CAD build for the part. Positions are in the model's coordinates, mm. Give positions to 0.01 mm unless a question says otherwise; leave off trailing zeros. Loops run counter-clockwise (first coordinate to the right, second up) from the corner with the lowest first, then second, coordinate; pieces in that order, holes last. Notation, with made-up numbers: M 71.25,37 L 87.25,37 A25 cw 87.25,73 Z; hole C 18.5,-18 d8. An arc over 180 degrees is marked long. Answer as CSV lines item,"result".
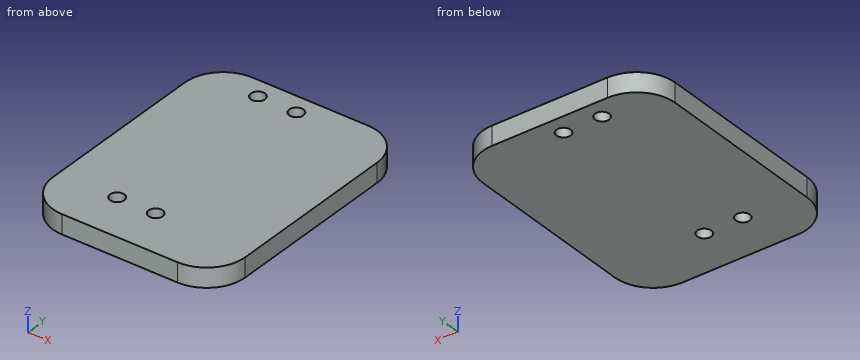
from build123d import *

# Parameters (mm, degrees)
ESQUISSE1_W             = 50
ESQUISSE1_H             = 65
BOSS_EXTRU_1_DEPTH      = 5
ESQUISSE2_R             = 1.85
ENL_V_MAT_EXTRU_1_DEPTH = 42.306779105
CONG_1_R                = 10


with BuildPart() as part:
    # Esquisse1 → Boss.-Extru.1 (new body)
    with BuildSketch(Plane.XY):
        Rectangle(ESQUISSE1_W, ESQUISSE1_H)
    extrude(amount=BOSS_EXTRU_1_DEPTH)

    # Esquisse2 → Enlèv. mat.-Extru.1 (cut, through all)
    with BuildSketch(Plane.XY.offset(5)):
        with Locations((-9.8, -20.5)):
            Circle(ESQUISSE2_R)
        with Locations((0.2, -20.5)):
            Circle(ESQUISSE2_R)
        with Locations((-9.8, 27.5)):
            Circle(ESQUISSE2_R)
        with Locations((0.2, 27.5)):
            Circle(ESQUISSE2_R)
    extrude(amount=-ENL_V_MAT_EXTRU_1_DEPTH, mode=Mode.SUBTRACT)

    # Congé1
    cong_1_edges = [part.edges().sort_by_distance(p)[0] for p in [
        (25, -32.5, 2.5),
        (-25, -32.5, 2.5),
        (-25, 32.5, 2.5),
        (25, 32.5, 2.5),
    ]]
    fillet(cong_1_edges, radius=CONG_1_R)


solid = part.part
1) Band-saw the part on C-C on z = 4.15. Give the cut face in (x, y), and give its area (3 significant figures).
Answer below:
outline,"M -25,-22.5 A10 ccw -15,-32.5 L 15,-32.5 A10 ccw 25,-22.5 L 25,22.5 A10 ccw 15,32.5 L -15,32.5 A10 ccw -25,22.5 Z; hole C -9.8,-20.5 d3.7; hole C -9.8,27.5 d3.7; hole C 0.2,-20.5 d3.7; hole C 0.2,27.5 d3.7"
area,"3,120 mm^2"
2) Band-saw the part on B-B on y = -20.5. Give the cut face in (x, z), and give its area (3 significant figures).
Answer below:
outline,"M -25,0 L -11.65,0 L -11.65,5 L -25,5 Z; M -7.95,0 L -1.65,0 L -1.65,5 L -7.95,5 Z; M 2.05,0 L 25,0 L 25,5 L 2.05,5 Z"
area,"213 mm^2"
3) Band-saw the part on A-A on x = 0.2. Give the cut face in (y, z), and give its area (3 significant figures).
Answer below:
outline,"M -32.5,0 L -22.35,0 L -22.35,5 L -32.5,5 Z; M -18.65,0 L 25.65,0 L 25.65,5 L -18.65,5 Z; M 29.35,0 L 32.5,0 L 32.5,5 L 29.35,5 Z"
area,"288 mm^2"
4) Flat gauge pin, fed straight in: pin 1 (3 mm diameter, centred on x = 0.2, y = 27.5, fed in from +Z) (1 decimal). Where does the tip first touch, or does it go through?
Answer below:
pin 1,"passes through"
5) Drill centre lines: line 1 (Y direction, x = -9.8, z = 2.35); line 2 (Y direction, x = -0.5, z = 3.4); line 3 (X direction, y = 23, z = 0.5). Where is each one in solid material? Low to high. Write a range as from..to.
Answer below:
line 1,"y = -32.5..-22.35, -18.65..25.65, 29.35..32.5"
line 2,"y = -32.5..-22.21, -18.79..25.79, 29.21..32.5"
line 3,"x = -24.99..24.99"
